```python
from build123d import *

# Parameters (mm, degrees)
SKETCH1_R                = 51.5
BOSS_EXTRUDE1_DEPTH      = 2.8
SKETCH2_R                = 51.302702975
SKETCH2_R_2              = 49
BOSS_EXTRUDE2_DEPTH      = 40
CUT_EXTRUDE1_DEPTH       = 2.8
SNAP_START               = -32.152970268
SNAP_GROOVE2_DEPTH       = 1.05
SNAP_START_2             = -33.102970268
SNAP_GROOVE2_2_DEPTH     = 0.95
CUT_EXTRUDE9_DEPTH       = 123.425444719
MIRROR10_START           = -32.152970268
MIRROR10_COPY_1_DEPTH    = 1.05
MIRROR10_START_2         = -33.102970268
MIRROR10_COPY_2_DEPTH    = 0.95
MIRROR10_COPY_3_DEPTH    = 0.95
SKETCH23_W               = 0.31
SKETCH23_H               = 8.321250797
CUT_EXTRUDE18_DEPTH      = 10
MIRROR12_COPY_1_SKETCH_W = 0.31
MIRROR12_COPY_1_SKETCH_H = 8.321250797
MIRROR12_COPY_1_DEPTH    = 10


# Read off the part's stored shape, not the designer's step: Snap Groove2
with BuildPart() as part:
    # Sketch1 → Boss-Extrude1 (new body)
    with BuildSketch(Plane(origin=(0, 0, 0), x_dir=(1, 0, 0), z_dir=(0, 1, 0))):
        with Locations(Location((0, 0, 0), (0, 0, 270))):
            Circle(SKETCH1_R)
    extrude(amount=BOSS_EXTRUDE1_DEPTH)

    # Sketch2 → Boss-Extrude2 (add)
    with BuildSketch(Plane(origin=(0, 2.8, 0), x_dir=(1, 0, 0), z_dir=(0, 1, 0))):
        with Locations(Location((0, 0, 0), (0, 0, 270))):
            Circle(SKETCH2_R)
        with Locations(Location((0, 0, 0), (0, 0, 270))):
            Circle(SKETCH2_R_2, mode=Mode.SUBTRACT)
    extrude(amount=BOSS_EXTRUDE2_DEPTH)

    # Sketch3 → Cut-Extrude1 (cut)
    with BuildSketch(Plane(origin=(0, 2.8, 0), x_dir=(1, 0, 0), z_dir=(0, 1, 0))):
        Polygon((28.803377941, 30.903803584), (28.803377941, -35.91647658), (22.504161148, -35.91647658), (22.611913195, -42.365053075), (21.509867104, -43.633319461), (18.751547007, -44.925112233), (17.307649543, -45.070983147), (-17.226935769, -45.070983147), (-18.600923478, -44.925112233), (-21.77353452, -43.416317025), (-21.77353452, -43.046957831), (-21.893563057, -35.863677115), (-28.534712584, -35.863677115), (-28.534712584, 31.993942871), (-21.893563057, 31.993942871), (-21.77353452, 40.794290055), (-21.388795882, 41.368785458), (22.021637567, 41.368785458), (22.058242529, 41.352489898), (22.058242529, 32.561962301), (28.803377941, 32.561962301), align=None)
    extrude(amount=-CUT_EXTRUDE1_DEPTH, mode=Mode.SUBTRACT)

    # Sketch5 → Revolve1 (revolve)
    with BuildSketch(Plane(origin=(0, 0, 0), x_dir=(0, 0, -1), z_dir=(1, 0, 0)), mode=Mode.PRIVATE) as revolve1_sk:
        with BuildLine():
            Line((-51.302702975, 42.8), (-49.053064555, 42.8))
            Line((-49.053064555, 42.8), (-49.053064555, 55.8))
            Line((-49.053064555, 55.8), (-60.053064555, 55.8))
            Line((-60.053064555, 55.8), (-60.053064555, 53.073629834))
            ThreePointArc((-60.053064555, 53.073629834), (-54.22806986, 49.171665315), (-51.302702975, 42.8))
        make_face()
        Polygon((-60.053064555, 53.073629834), (-60.053064555, 55.8), (-62.053064555, 55.8), (-62.053064555, 52.983272883), (-60.053064555, 52.983272883), align=None)
        with BuildLine():
            Line((-62.053064555, 52.983272883), (-62.053064555, 55.8))
            Line((-62.053064555, 55.8), (-73.053064555, 55.8))
            Line((-73.053064555, 55.8), (-73.053064555, 53.073629834))
            ThreePointArc((-73.053064555, 53.073629834), (-67.22806986, 49.171665315), (-64.302702975, 42.8))
            Line((-64.302702975, 42.8), (-62.053064555, 42.8))
            Line((-62.053064555, 42.8), (-62.053064555, 52.983272883))
        make_face()
        Polygon((-73.053064555, 53.073629834), (-73.053064555, 55.8), (-77.053064555, 55.8), (-77.053064555, 41.8), (-75.053064555, 41.8), (-75.053064555, 52.983272883), (-73.053064555, 52.983272883), align=None)
    revolve(revolve1_sk.sketch.rotate(Axis((0, 42.8, 0), (0, 1, 0)), 180), axis=Axis((0, 42.8, 0), (0, 1, 0)))

    # Snap Groove2 outline → Snap Groove2 (cut)
    with BuildSketch(Plane.YZ.offset(SNAP_START)):
        Polygon((0, 7.425343804), (0, 1.722535804), (2.8, 0.416874361), (2.8, 8.731005247), align=None)
    snap_groove2 = extrude(amount=SNAP_GROOVE2_DEPTH, mode=Mode.SUBTRACT)

    # Snap Groove2 2 outline → Snap Groove2 2 (cut)
    with BuildSketch(Plane.YZ.offset(SNAP_START_2)):
        Polygon((0, 7.425343804), (0, 1.722535804), (0.54641169, 1.467739849), (0.54641169, 7.68013976), align=None)
    snap_groove2_2 = extrude(amount=SNAP_GROOVE2_2_DEPTH, mode=Mode.SUBTRACT)

    # Sketch13 → Cut-Extrude9 (cut, symmetric)
    with BuildSketch(Plane(origin=(0, 55.8, 0), x_dir=(1, 0, 0), z_dir=(0, 1, 0))):
        Polygon((-92.348219575, -56.21042489), (-92.348219575, 56.21042489), (-52.702589035, 56.21042489), (-33.965663886, 35.317611426), (-33.965663886, -35.317611426), (-52.702589035, -56.21042489), align=None)
    cut_extrude9 = extrude(amount=CUT_EXTRUDE9_DEPTH, both=True, mode=Mode.SUBTRACT)

    # Mirror7: Cut-Extrude9 across plane
    add(cut_extrude9.mirror(Plane(origin=(0, 0, 0), x_dir=(0, 0, 1), z_dir=(1, 0, 0))), mode=Mode.SUBTRACT)

    # Mirror9: Snap Groove2, Snap Groove2 2 across plane
    add(snap_groove2.mirror(Plane(origin=(0, 0, 0), x_dir=(0, 0, 1), z_dir=(1, 0, 0))), mode=Mode.SUBTRACT)
    add(snap_groove2_2.mirror(Plane(origin=(0, 0, 0), x_dir=(0, 0, 1), z_dir=(1, 0, 0))), mode=Mode.SUBTRACT)

    # Mirror10: Snap Groove2, Snap Groove2 2 across plane
    add(snap_groove2.mirror(Plane(origin=(0.02272558, 10.52276449, -10.082239745), x_dir=(1, 0, 0), z_dir=(0, 0, -1))), mode=Mode.SUBTRACT)
    add(snap_groove2_2.mirror(Plane(origin=(0.02272558, 10.52276449, -10.082239745), x_dir=(1, 0, 0), z_dir=(0, 0, -1))), mode=Mode.SUBTRACT)

    # Mirror10 copy 1 sketch → Mirror10 copy 1 (cut)
    with BuildSketch(Plane(origin=(0, 0, -20.164479489), x_dir=(0, 1, 0), z_dir=(-1, 0, 0)).offset(MIRROR10_START)):
        Polygon((0, 7.425343804), (0, 1.722535804), (2.8, 0.416874361), (2.8, 8.731005247), align=None)
    extrude(amount=MIRROR10_COPY_1_DEPTH, mode=Mode.SUBTRACT)

    # Mirror10 copy 2 sketch → Mirror10 copy 2 (cut)
    with BuildSketch(Plane(origin=(0, 0, -20.164479489), x_dir=(0, 1, 0), z_dir=(-1, 0, 0)).offset(MIRROR10_START_2)):
        Polygon((0, 7.425343804), (0, 1.722535804), (0.54641169, 1.467739849), (0.54641169, 7.68013976), align=None)
    extrude(amount=MIRROR10_COPY_2_DEPTH, mode=Mode.SUBTRACT)

    # Mirror10 copy 3 sketch → Mirror10 copy 3 (cut)
    with BuildSketch(Plane(origin=(0, 0, -20.164479489), x_dir=(0, 1, 0), z_dir=(1, 0, 0)).offset(MIRROR10_START_2)):
        Polygon((0, -7.425343804), (0, -1.722535804), (0.54641169, -1.467739849), (0.54641169, -7.68013976), align=None)
    extrude(amount=MIRROR10_COPY_3_DEPTH, mode=Mode.SUBTRACT)

    # Sketch23 → Cut-Extrude18 (cut)
    with BuildSketch(Plane(origin=(0, 2.8, 0), x_dir=(1, 0, 0), z_dir=(0, 1, 0))):
        with Locations((30.947970268, 24.74197925)):
            Rectangle(SKETCH23_W, SKETCH23_H)
    cut_extrude18 = extrude(amount=-CUT_EXTRUDE18_DEPTH, mode=Mode.SUBTRACT)

    # Mirror11: Cut-Extrude18 across plane
    add(cut_extrude18.mirror(Plane(origin=(0, 0, 0), x_dir=(0, 0, 1), z_dir=(1, 0, 0))), mode=Mode.SUBTRACT)

    # Mirror12: Cut-Extrude18 across plane
    add(cut_extrude18.mirror(Plane(origin=(0.02272558, 10.52276449, -10.082239745), x_dir=(1, 0, 0), z_dir=(0, 0, -1))), mode=Mode.SUBTRACT)

    # Mirror12 copy 1 sketch → Mirror12 copy 1 (cut)
    with BuildSketch(Plane(origin=(0, 2.8, -20.164479489), x_dir=(-1, 0, 0), z_dir=(0, 1, 0))):
        with Locations((30.947970268, 24.74197925)):
            Rectangle(MIRROR12_COPY_1_SKETCH_W, MIRROR12_COPY_1_SKETCH_H)
    extrude(amount=-MIRROR12_COPY_1_DEPTH, mode=Mode.SUBTRACT)


solid = part.part
```
The listing builds one solid part. Answer for the finished solid, in the listing's coordinates (mm). A direction names the side the tool comes from. Coordinates: 2 decimals unless noted, no trailing zeros. Write each loop counter-clockwise with the first axis right and the second up, starting at its lowest first coordinate (ties: lowest second). Pieces come first, ordered by that corner, then holes. Notation, with made-up numbers: (28, 80) -> (36, 80) arc R17 ccw to (36, 103) -> close; hole circle Ø6 at (34.5, 27.5). An arc over 180 degrees is marked (long way). Write each question's results on one line, items separated by ' | '. Start each with the question number.
1) Flat-ended cylindrical pins translate along their axes: pin 1 Ø3 at (x, y) = (-22.5, 11) entering from -Z; pin 2 Ø8 at (x, y) = (8, 21) entering from +Z; pin 3 Ø1.1 at (y, z) = (1, 6) entering from +X. Find the tip coordinate at first contact, or state that the pin passes through.
2) A tool of negligible diameter and unlimited length cuts with its end or side. For faces 1 (the flat face through (-4, 41.8, -76)), 2 (the cylindrical face through (-0.551, 1.38, 51.497)), 3 (the cylindrical face through (0.81, 48.7, -77.05)), 4 (the flat face through (-43.378, 44.564, -45.813)), 5 (the flat face through (-0.2, 52.983, -60.3)), from which of +Z, -Z, +X, -X, +Y, -Y can it reach the whole face along a straight path? Write none if from no direction.
3) Straight lines are drawn through the part: probe 1 along X at (y, z) = (2, 32.5); probe 2 along Z at (x, y) = (-5.5, 48.5); probe 3 along Y at (x, z) = (-32.5, -8.5). For each, find the intervals that lie inside material, in ascending order.
4) For a pull along Y with two mould halves and no side action, classify faces 6 (the flat face through (-30, 2.8, -7)), 7 (the cylindrical face through (-0.5, 22.5, 51.3)), 8 (the flat face through (0, 41.8, 76)), 9 (the flat face through (43.29, 44.564, 45.715)) as +Y half, -Y half, draft (parallel to the pull), parting line (faces both ways), or undercut.
5) A cutting plane is placed at A-A (y = 14). Determine the outline of the cut face in (x, z).
6) A cutting plane is placed at C-C (y = 48.5). Determine the outline of the cut face in (x, z).
7) A cutting plane is placed at B-B (z = 15). Determine the outline of the cut face in (x, y), then the cut area to 3 significant figures.
Values follow:
1) pin 1: z = -46.81 | pin 2: z = 51.15 | pin 3: x = 33.97
2) face 1: -Z, +X, -X, -Y | face 2: +Z, -Y | face 3: -Z, +Y, -Y | face 4: -X, +Y, -Y | face 5: -Y
3) probe 1: -33.97 to -28.53, 28.8 to 33.97 | probe 2: -76.86 to -74.85, -66.47 to -61.81, -53.41 to -48.74, 48.74 to 53.41, 61.81 to 66.47, 74.85 to 76.86 | probe 3: 0 to 2.8
4) face 6: +Y half | face 7: undercut | face 8: -Y half | face 9: draft
5) outline: (-35.5, -37.03) arc R51.3 ccw to (35.5, -37.03) -> (33.97, -35.32) arc R49 cw to (-33.97, -35.32) -> close; (-35.5, 37.03) -> (-33.97, 35.32) arc R49 cw to (33.97, 35.32) -> (35.5, 37.03) arc R51.3 ccw to start
6) outline: (-52.7, -56.21) arc R77.05 ccw to (52.7, -56.21) -> (51.37, -54.72) arc R75.05 cw to (-51.37, -54.72) -> close; (-52.7, 56.21) -> (-51.37, 54.72) arc R75.05 cw to (51.37, 54.72) -> (52.7, 56.21) arc R77.05 ccw to start; (-45.78, -48.5) arc R66.69 ccw to (45.78, -48.5) -> (42.68, -45.04) arc R62.05 cw to (-42.68, -45.04) -> close; (-45.78, 48.5) -> (-42.68, 45.04) arc R62.05 cw to (42.68, 45.04) -> (45.78, 48.5) arc R66.69 ccw to start; (-37.1, -38.81) arc R53.69 ccw to (37.1, -38.81) -> (34, -35.36) arc R49.05 cw to (-34, -35.36) -> close; (-37.1, 38.81) -> (-34, 35.36) arc R49.05 cw to (34, 35.36) -> (37.1, 38.81) arc R53.69 ccw to start
7) outline: (-33.97, 0) -> (-28.53, 0) -> (-28.53, 2.8) -> (-33.97, 2.8) -> close; (28.8, 0) -> (33.97, 0) -> (33.97, 2.8) -> (28.8, 2.8) -> close | area: 29.7 mm²
